Design review of the part built by this model. Coordinates are the model's own, in mm. Face numbers are marked on the shaded views. A direction names the side the tool comes from. Coordinates: 2 decimals unless noted, no trailing zeros. Loops run counter-clockwise (first coordinate to the right, second up) from the corner with the lowest first, then second, coordinate; pieces in that order, holes last. Notation, with made-up numbers: M 45,46 L 74,46 A30 cw 74,71 Z; hole C -32.75,23 d9. An arc over 180 degrees is marked long. Put each result on its own line as item: value. Start each with the question number.
(1) Clearance check with flat-ended pins moving along their axes: pin 1 (4.5 mm diameter, centred on x = 0, y = 27.5, fed in from -Z); pin 2 (1.5 mm diameter, centred on y = 16, z = 10, fed in from +X); pin 3 (1.5 mm diameter, centred on y = 5, z = 3, fed in from +X); pin 4 (10 mm diameter, centred on x = 22.5, z = 9, fed in from +Y). State where each tip first meets the part, or that it passes through.
(2) Take a section at B-B, the plane y = 13. Give the boundary of the cut face in (x, z).
(3) The part is to be moulded in two halves that separate along Y. For the marked faces 1, 2 and 3, say which applies: +Y half, -Y half, draft (parallel to the pull), parting line (faces both ways), or undercut.
(4) For probe 1 along X at (y, z) = (17.5, 2.75); probe 2 along X at (y, z) = (-3.5, 6.5); probe 3 along Y at (x, z) = (0, 6.5), list the stretches that pass through material, from the lowest coordinate up. Write a range as [from, to].
(5) Take a section at D-D, the plane z = 6.5. Give the boundary of the cut face in (x, y), then the cut area to 3 significant figures.
(6) Take a section at C-C, the plane y = 18.5. Give the boundary of the cut face in (x, z).
(7) Take a section at A-A, the plane x = 0. Give the boundary of the cut face in (y, z), then the cut area to 3 significant figures.
(8) For the marked faces 4 and 5, list the 3-axis set-ups (+Z, -Z, +X, -X, +Y, -Y) from which the entire face can be reached by the end or side of a thin tool; tool diameter is ignored.
```python
from build123d import *

# Parameters (mm, degrees)
EXTRUDE_1_DEPTH          = 18
CUT_EXTRUDE_1_DEPTH      = 19
HOLE_WIZARD_M4_2_D       = 4.8
PATTERN_CIRCULAR_1_COUNT = 8


with BuildPart() as part:
    # ｽｹｯﾁ1 → ﾎﾞｽ - 押し出し1 (new body)
    with BuildSketch(Plane.XY):
        with BuildLine():
            ThreePointArc((-31, 0), (0, 31), (31, 0))
            Line((31, 0), (31, -11))
            Line((31, -11), (-31, -11))
            Line((-31, -11), (-31, 0))
        make_face()
    extrude(amount=EXTRUDE_1_DEPTH)

    # ｽｹｯﾁ2 → ｶｯﾄ - 押し出し1 (cut, through all)
    with BuildSketch(Plane.XY.offset(18)):
        with BuildLine():
            Line((-24, 0), (-24, -11))
            Line((-24, -11), (24, -11))
            Line((24, -11), (24, 0))
            ThreePointArc((24, 0), (0, 24), (-24, 0))
        make_face()
    extrude(amount=-CUT_EXTRUDE_1_DEPTH, mode=Mode.SUBTRACT)

    # M4 すきま穴2 (through all)
    with Locations(Plane.XY.offset(18)):
        with Locations((0, 27.5)):
            hole_wizard_m4_2 = Hole(HOLE_WIZARD_M4_2_D / 2)

    # 円形ﾊﾟﾀｰﾝ1: M4 すきま穴2 ×8 about axis, 3 skipped
    pattern_circular_1_axis = Axis((0, 0, 0), (0, 0, -1))
    add([hole_wizard_m4_2.rotate(pattern_circular_1_axis, i * 360 / PATTERN_CIRCULAR_1_COUNT) for i in range(1, PATTERN_CIRCULAR_1_COUNT) if i not in (3, 4, 5)], mode=Mode.SUBTRACT)


solid = part.part
```
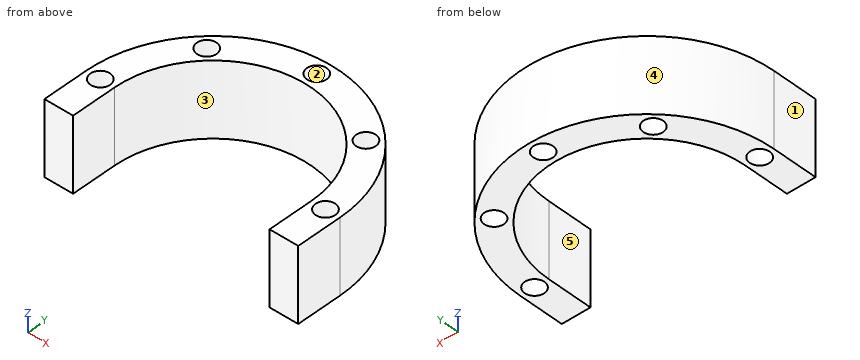
Computed values:
1. pin 1: passes through
1. pin 2: stops at x = 26.99
1. pin 3: stops at x = 30.71
1. pin 4: stops at y = 25.59
2. outline: M -28.14,0 L -20.17,0 L -20.17,18 L -28.14,18 Z; M 20.17,0 L 28.14,0 L 28.14,18 L 20.17,18 Z
3. face 1: draft
3. face 2: undercut
3. face 3: -Y half
4. probe 1: x = [-25.59, -20.85], [-18.04, -16.42], [16.42, 18.04], [20.85, 25.59]
4. probe 2: x = [-31, -24], [24, 31]
4. probe 3: y = [24, 25.1], [29.9, 31]
5. outline: M -31,-11 L -24,-11 L -24,0 A24 cw 24,0 L 24,-11 L 31,-11 L 31,0 A31 ccw -31,0 Z; hole C -27.5,0 d4.8; hole C -19.45,19.45 d4.8; hole C 0,27.5 d4.8; hole C 19.45,19.45 d4.8; hole C 27.5,0 d4.8
5. area: 668 mm^2
6. outline: M -24.87,0 L -21.65,0 L -21.65,18 L -24.87,18 Z; M -17.24,0 L -15.29,0 L -15.29,18 L -17.24,18 Z; M 15.29,0 L 17.24,0 L 17.24,18 L 15.29,18 Z; M 21.65,0 L 24.87,0 L 24.87,18 L 21.65,18 Z
7. outline: M 24,0 L 25.1,0 L 25.1,18 L 24,18 Z; M 29.9,0 L 31,0 L 31,18 L 29.9,18 Z
7. area: 39.6 mm^2
8. face 4: +Z, -Z, +Y
8. face 5: +Z, -Z, -Y
